from build123d import *

# Parameters (mm, degrees)
SKETCH2_W       = 41.253356914
SKETCH2_H       = 34.3662
SKETCH2_R       = 3.2639
MAIN_BODY_DEPTH = 2.54
FILLET1_R       = 3.175
SKETCH3_W       = 6.5278
SKETCH3_H       = 17.1831
SLOTS_DEPTH     = 27.966097044


with BuildPart() as part:
    # Sketch2 → Main Body (new body)
    with BuildSketch(Plane(origin=(0, 0, 0), x_dir=(1, 0, 0), z_dir=(0, 1, 0))):
        Rectangle(SKETCH2_W, SKETCH2_H)
        with Locations(Location((-13.006678457, 0, 0), (0, 0, 270))):
            Circle(SKETCH2_R, mode=Mode.SUBTRACT)
        with Locations(Location((13.006678457, 0, 0), (0, 0, 90))):
            Circle(SKETCH2_R, mode=Mode.SUBTRACT)
    extrude(amount=MAIN_BODY_DEPTH)

    # Fillet1
    fillet1_edges = [part.edges().sort_by_distance(p)[0] for p in [
        (20.626678457, 1.27, 17.1831),
        (-20.626678457, 1.27, 17.1831),
    ]]
    fillet(fillet1_edges, radius=FILLET1_R)

    # Sketch3 → Slots (cut, through all)
    with BuildSketch(Plane(origin=(0, 2.54, 0), x_dir=(1, 0, 0), z_dir=(0, 1, 0))):
        with Locations((-13.006678457, 8.59155)):
            Rectangle(SKETCH3_W, SKETCH3_H)
        with Locations((13.006678457, 8.59155)):
            Rectangle(SKETCH3_W, SKETCH3_H)
    extrude(amount=-SLOTS_DEPTH, mode=Mode.SUBTRACT)


solid = part.part
For this review, take the finished solid that the model builds, in its own axes (mm). A direction names the side the tool comes from. Give positions to 0.01 mm unless a question says otherwise; leave off trailing zeros. Write each loop counter-clockwise with the first axis right and the second up, starting at its lowest first coordinate (ties: lowest second). Pieces come first, ordered by that corner, then holes. Notation, with made-up numbers: (18.25, 0.25) -> (64.25, 0.25) arc R12 cw to (64.25, 4.25) -> close; hole circle Ø3 at (58.5, 14.5). An arc over 180 degrees is marked (long way). Use CSV: the item, a comma, the result in double quotes.
Q1. To check wall thickness, follow probe 1 along X at (y, z) = (1.85, -9.5); probe 2 along X at (y, z) = (1.6, 3); probe 3 along Z at (x, y) = (18.5, 1.85). State the ranges of each line that lie inside material, in increasing order. Write a range as [from, to].
Conclusion:
probe 1,"[-20.63, -16.27], [-9.74, 9.74], [16.27, 20.63]"
probe 2,"[-20.63, -14.29], [-11.72, 11.72], [14.29, 20.63]"
probe 3,"[-17.18, 17.01]"
Q2. Take a section at C-C, the plane x = -13. Write out the cut boundary in (y, z).
Conclusion:
outline,"(0, 3.26) -> (2.54, 3.26) -> (2.54, 17.18) -> (0, 17.18) -> close"
Q3. Mouldability with a two-part tool opening along X and no side actions: class faces 1 (the face through (9.743, 1, -8)), 2 (the face through (-19.72, 1.29, 16.23)), 3 (the face through (0, 1, 17.183)), 4 (the face through (-9.743, 1, -8)) as pulls with the +X half, pulls with the -X half, needs draft (parallel to the pull), parting line crosses it, or undercut.
Conclusion:
face 1,"undercut"
face 2,"pulls with the -X half"
face 3,"needs draft"
face 4,"undercut"
Q4. Take a section at B-B, the plane y = 1.8. Write out the cut boundary in (x, z) (3 decimals), then the cut area to 3 significant figures.
Conclusion:
outline,"(-20.627, -17.183) -> (-16.271, -17.183) -> (-16.271, 0) arc R3.264 cw to (-9.743, 0) -> (-9.743, -17.183) -> (9.743, -17.183) -> (9.743, 0) arc R3.264 cw to (16.271, 0) -> (16.271, -17.183) -> (20.627, -17.183) -> (20.627, 14.008) arc R3.175 ccw to (17.452, 17.183) -> (-17.452, 17.183) arc R3.175 ccw to (-20.627, 14.008) -> close"
area,"1,160 mm2"
Q5. Take a section at A-A, the plane z = -0.5. Write out the cut boundary in (x, y), then the cut area to 3 significant figures.
Conclusion:
outline,"(-20.63, 0) -> (-16.27, 0) -> (-16.27, 2.54) -> (-20.63, 2.54) -> close; (-9.74, 0) -> (9.74, 0) -> (9.74, 2.54) -> (-9.74, 2.54) -> close; (16.27, 0) -> (20.63, 0) -> (20.63, 2.54) -> (16.27, 2.54) -> close"
area,"71.6 mm2"
Q6. Tool access review of faces 5 (the face through (16.271, 1, -8)), 6 (the face through (20.627, 1, -1)): name each direction out of +Z, -Z, +X, -X, +Y, -Y from which nothing blocks a thin tool from reaching the whole face with its end or side.
Conclusion:
face 5,"-Z, +Y, -Y"
face 6,"+Z, -Z, +X, +Y, -Y"
